Could you check a few things on this model? Use its own coordinates, in mm. Give positions to 0.01 mm unless a question says otherwise; leave off trailing zeros. Order: outer loops, then holes, each group sorted by start corner. A loop starts at its lowest first (then second) coordinate and runs counter-clockwise, first axis right, second up. Notation, with made-up numbers: (38, 89) - (58, 89) arc R32 cw to (58, 118) - close; hole circle Ø8 at (50.5, 3.25). An arc over 180 degrees is marked (long way). One line per question, with ' | ' between items. Start each with the question number.
1. I need wall thicknesses on probe 1 along Y at (x, z) = (-21, 2.2) (3 decimals); probe 2 along X at (y, z) = (6.5, 0.95); probe 3 along X at (y, z) = (-14, 1.05) (3 decimals). Which ranges of each line are inside material? Lowest first, please. Write a range as from..to.
2. Imagine slicing it at C-C (z = 1.2). Give the number of separate pieces and of enclosed holes in the cut face, and give its area (3 significant figures).
3. Imagine slicing it at B-B (y = -2). Please give me the cut outline in (x, z) (3 decimals).
4. Imagine slicing it at A-A (x = 12.5). Please give me the cut outline in (y, z) (3 decimals).
5. For P1, Ø1.4, axis at x = 58, z = 1, coming from the +Y side; P2, Ø1.4, axis at x = 58, z = 2, coming from the -Y side; P3, Ø1.2, axis at y = 15.5, z = 2, coming from the -X side; P4, Ø4, axis at x = 23, y = 8, coming from the -Z side, each with a flat end and sliding along its axis, tell me the tip position at first contact or that it passes through.
```python
from build123d import *

# Parameters (mm, degrees)
SKETCH1_W           = 124.35
SKETCH1_H           = 33
BOSS_EXTRUDE1_DEPTH = 3.175
SKETCH2_W           = 9.65
SKETCH2_H           = 2.8
SKETCH2_H_2         = 3
CUT_EXTRUDE1_DEPTH  = 65.405444257
SKETCH4_W           = 2.8
SKETCH4_H           = 3
SKETCH4_W_2         = 6.175
SKETCH4_H_2         = 15
CUT_EXTRUDE2_DEPTH  = 65.405444257
SKETCH6_W           = 3
SKETCH6_H           = 1.375
CUT_EXTRUDE3_DEPTH  = 65.405444257
CUT_SWEEP1_DEPTH    = 3.175
SKETCH12_R          = 0.75
CUT_EXTRUDE6_DEPTH  = 65.405444385
CUT_EXTRUDE7_DEPTH  = 65.405444385
FILLET6_R           = 2
FILLET7_R           = 0.5
SKETCH15_W          = 20
SKETCH15_H          = 16
CUT_EXTRUDE9_DEPTH  = 65.405444385
FILLET9_R           = 0.5


# Read off the part's stored shape, not the designer's step: Cut-Sweep1
with BuildPart() as part:
    # Sketch1 → Boss-Extrude1 (new body)
    with BuildSketch(Plane.XY):
        Rectangle(SKETCH1_W, SKETCH1_H)
    extrude(amount=BOSS_EXTRUDE1_DEPTH)

    # Sketch2 → Cut-Extrude1 (cut, through all)
    with BuildSketch(Plane.XY.offset(3.175)):
        with Locations((-25, -13.1)):
            Rectangle(SKETCH2_W, SKETCH2_H)
        with Locations((25, -13.1)):
            Rectangle(SKETCH2_W, SKETCH2_H)
        with Locations((-25, 15)):
            Rectangle(SKETCH2_W, SKETCH2_H_2)
        with Locations((25, 15)):
            Rectangle(SKETCH2_W, SKETCH2_H_2)
    extrude(amount=-CUT_EXTRUDE1_DEPTH, mode=Mode.SUBTRACT)

    # Sketch4 → Cut-Extrude2 (cut, through all)
    with BuildSketch(Plane.XY.offset(3.175)):
        with Locations((-57.775, 15)):
            Rectangle(SKETCH4_W, SKETCH4_H)
        with Locations((-59.0875, 0)):
            Rectangle(SKETCH4_W_2, SKETCH4_H_2)
        with Locations((-57.775, -15)):
            Rectangle(SKETCH4_W, SKETCH4_H)
        with Locations((57.775, 15)):
            Rectangle(SKETCH4_W, SKETCH4_H)
        with Locations((59.0875, 0)):
            Rectangle(SKETCH4_W_2, SKETCH4_H_2)
        with Locations((57.775, -15)):
            Rectangle(SKETCH4_W, SKETCH4_H)
    extrude(amount=-CUT_EXTRUDE2_DEPTH, mode=Mode.SUBTRACT)

    # Sketch6 → Cut-Extrude3 (cut, through all)
    with BuildSketch(Plane.XY.offset(3.175)):
        with Locations((-60.675, 15.8125)):
            Rectangle(SKETCH6_W, SKETCH6_H)
        with Locations((-60.675, -15.8125)):
            Rectangle(SKETCH6_W, SKETCH6_H)
        with Locations((60.675, 15.8125)):
            Rectangle(SKETCH6_W, SKETCH6_H)
        with Locations((60.675, -15.8125)):
            Rectangle(SKETCH6_W, SKETCH6_H)
    extrude(amount=-CUT_EXTRUDE3_DEPTH, mode=Mode.SUBTRACT)

    # Cut-Sweep1 outline → Cut-Sweep1 (cut)
    with BuildSketch(Plane.XY):
        with BuildLine():
            add(Edge.make_bspline(
                [(-56, -6), (-55.016272395, -6.040912607), (-53.484317245, -6.110006936), (-52.10462272, -6.208217255), (-51.370216858, -6.312882143), (-50.849013323, -6.424427059), (-50.274077583, -6.562740427), (-49.507561658, -6.770408498), (-47.98416767, -7.234467607), (-46.535590196, -7.742954919), (-44.899823838, -8.383891144), (-43.265010906, -9.091671777), (-41.074137026, -10.055384808), (-38.357692762, -10.850187014), (-36.1078612, -11.027108547), (-34.793437631, -10.999002823)],
                knots=[0, 0, 0, 0, 0.052266667, 0.104533333, 0.1568, 0.188540911, 0.209066667, 0.261333333, 0.3136, 0.4368, 0.46346514, 0.56, 0.706666667, 0.853333333, 1, 1, 1, 1], degree=3))
            Line((-56, -6), (-56, -7.5))
            add(Edge.make_bspline(
                [(-56, -7.5), (-55.020423649, -7.540842864), (-53.496771007, -7.609797709), (-52.171479553, -7.70829789), (-51.569513747, -7.80075633), (-51.115986388, -7.900930823), (-50.592043829, -8.028791809), (-49.863497697, -8.22781936), (-48.398796638, -8.676488924), (-46.992197023, -9.172450468), (-45.412650318, -9.7933523), (-43.831176536, -10.480660701), (-41.561928867, -11.478467634), (-38.556226285, -12.350501385), (-36.110914304, -12.525218982), (-34.698750526, -12.49601129)],
                knots=[0, 0, 0, 0, 0.052266667, 0.104533333, 0.1568, 0.188540911, 0.209066667, 0.261333333, 0.3136, 0.4368, 0.46346514, 0.56, 0.706666667, 0.853333333, 1, 1, 1, 1], degree=3))
            Line((-34.698750526, -12.49601129), (-34.793437631, -10.999002823))
        make_face()
    cut_sweep1 = extrude(amount=CUT_SWEEP1_DEPTH, mode=Mode.SUBTRACT)

    # Mirror1: Cut-Sweep1 across plane
    add(cut_sweep1.mirror(Plane.ZY), mode=Mode.SUBTRACT)

    # Sketch12 → Cut-Extrude6 (cut, through all)
    with BuildSketch(Plane.XY.offset(3.175)):
        with Locations((-34.746094079, -11.747507056)):
            Circle(SKETCH12_R)
        with Locations((34.746094079, -11.747507056)):
            Circle(SKETCH12_R)
    extrude(amount=-CUT_EXTRUDE6_DEPTH, mode=Mode.SUBTRACT)

    # Sketch13 → Cut-Extrude7 (cut, through all)
    with BuildSketch(Plane.XY.offset(3.175)):
        Polygon((-56, 7.5), (-62.175, 11.3125), (-62.175, 7.5), align=None)
        Polygon((-56, -7.5), (-62.175, -11.3125), (-62.175, -7.5), align=None)
        Polygon((56, 7.5), (62.175, 11.3125), (62.175, 7.5), align=None)
        Polygon((56, -7.5), (62.175, -11.3125), (62.175, -7.5), align=None)
    extrude(amount=-CUT_EXTRUDE7_DEPTH, mode=Mode.SUBTRACT)

    # Fillet6
    fillet6_edges = [part.edges().sort_by_distance(p)[0] for p in [
        (62.175, -15.125, 1.5875),
        (62.175, -11.3125, 1.5875),
        (56, -7.5, 1.5875),
        (56, 7.5, 1.5875),
        (62.175, 11.3125, 1.5875),
        (62.175, 15.125, 1.5875),
        (-62.175, -15.125, 1.5875),
        (-62.175, -11.3125, 1.5875),
        (-56, -7.5, 1.5875),
        (-62.175, 15.125, 1.5875),
        (-62.175, 11.3125, 1.5875),
        (-56, 7.5, 1.5875),
    ]]
    fillet(fillet6_edges, radius=FILLET6_R)

    # Fillet7
    fillet7_edges = [part.edges().sort_by_distance(p)[0] for p in [
        (59.175, 15.125, 1.5875),
        (59.175, -15.125, 1.5875),
        (-59.175, -15.125, 1.5875),
        (-59.175, 15.125, 1.5875),
        (20.175, 16.5, 1.5875),
        (29.825, 16.5, 1.5875),
        (-20.175, 16.5, 1.5875),
        (-29.825, 16.5, 1.5875),
        (56.375, -16.5, 1.5875),
        (56, -6, 1.5875),
        (56.375, 16.5, 1.5875),
        (-56.375, 16.5, 1.5875),
        (-56.375, -16.5, 1.5875),
        (-56, -6, 1.5875),
    ]]
    fillet(fillet7_edges, radius=FILLET7_R)

    # Sketch15 → Cut-Extrude9 (cut, through all)
    with BuildSketch(Plane.XY.offset(3.175)):
        with Locations((-19, 3.275)):
            Rectangle(SKETCH15_W, SKETCH15_H)
        with Locations((19, 3.275)):
            Rectangle(SKETCH15_W, SKETCH15_H)
    extrude(amount=-CUT_EXTRUDE9_DEPTH, mode=Mode.SUBTRACT)

    # Fillet9
    fillet9_edges = [part.edges().sort_by_distance(p)[0] for p in [
        (-29, -4.725, 1.5875),
        (-29, 11.275, 1.5875),
        (-9, 11.275, 1.5875),
        (-9, -4.725, 1.5875),
        (9, -4.725, 1.5875),
        (9, 11.275, 1.5875),
        (29, 11.275, 1.5875),
        (29, -4.725, 1.5875),
    ]]
    fillet(fillet9_edges, radius=FILLET9_R)


solid = part.part
```
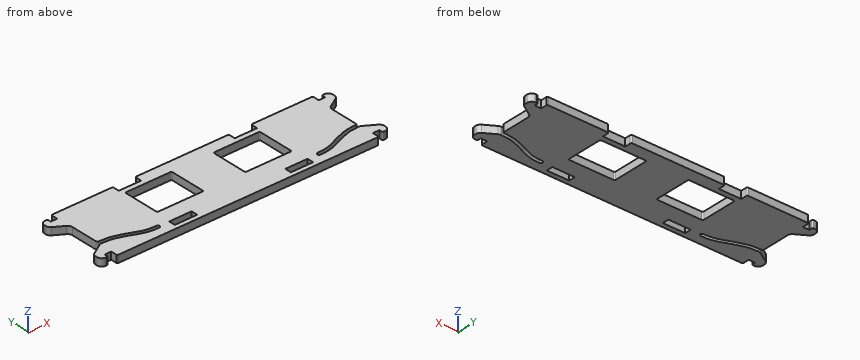
Results found:
1) probe 1: y = -16.5..-14.5, -11.7..-4.725, 11.275..13.5 | probe 2: x = -56..-29, -9..9, 29..56 | probe 3: x = -61.973..-59.175, -56.375..-29.825, -20.175..20.175, 29.825..56.375, 59.175..61.973
2) separate pieces: 1 | enclosed holes: 4 | area: 3,000 mm2
3) outline: (-56, 0) - (-29, 0) - (-29, 3.175) - (-56, 3.175) - close; (-9, 0) - (9, 0) - (9, 3.175) - (-9, 3.175) - close; (29, 0) - (56, 0) - (56, 3.175) - (29, 3.175) - close
4) outline: (-16.5, 0) - (-4.725, 0) - (-4.725, 3.175) - (-16.5, 3.175) - close; (11.275, 0) - (16.5, 0) - (16.5, 3.175) - (11.275, 3.175) - close
5) P1: stops at y = 13.5 | P2: stops at y = -13.5 | P3: stops at x = -61.1 | P4: passes through
